Can you work these out from the model? Positions are in its coordinate system, mm. Face numbers are marked on the shaded views. A direction names the side the tool comes from. Coordinates: 2 decimals unless noted, no trailing zeros. Order: outer loops, then holes, each group sorted by start corner. A loop starts at its lowest first (then second) coordinate and runs counter-clockwise, first axis right, second up. Notation, with made-up numbers: (-8.75, -16) -> (-2.75, -16) arc R21 cw to (-2.75, 18) -> close; hole circle Ø1 at (51.5, 2.25). An arc over 180 degrees is marked (long way). Write item = value, one per line.
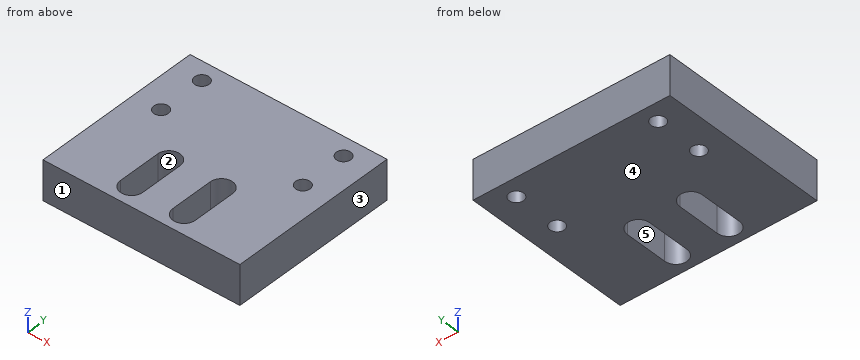
```python
from build123d import *

# Parameters (mm, degrees)
SKETCH1_W           = 75
SKETCH1_H           = 65
SKETCH1_R           = 2.75
BOSS_EXTRUDE1_DEPTH = 15


with BuildPart() as part:
    # Sketch1 → Boss-Extrude1 (new body)
    with BuildSketch(Plane.XY):
        with Locations((0, 1.421243981)):
            Rectangle(SKETCH1_W, SKETCH1_H)
        with Locations((-27, 8.921243981)):
            Circle(SKETCH1_R, mode=Mode.SUBTRACT)
        with Locations((-27, 26.921243981)):
            Circle(SKETCH1_R, mode=Mode.SUBTRACT)
        with Locations((27, 26.921243981)):
            Circle(SKETCH1_R, mode=Mode.SUBTRACT)
        with Locations((27, 8.921243981)):
            Circle(SKETCH1_R, mode=Mode.SUBTRACT)
        with BuildLine():
            Line((-5.75, -7.328756019), (-5.75, -23.828756019))
            ThreePointArc((-5.75, -23.828756019), (-10, -28.078756019), (-14.25, -23.828756019))
            Line((-14.25, -23.828756019), (-14.25, -7.328756019))
            ThreePointArc((-14.25, -7.328756019), (-10, -3.078756019), (-5.75, -7.328756019))
        make_face(mode=Mode.SUBTRACT)
        with BuildLine():
            Line((14.25, -7.328756019), (14.25, -23.828756019))
            ThreePointArc((14.25, -23.828756019), (10, -28.078756019), (5.75, -23.828756019))
            Line((5.75, -23.828756019), (5.75, -7.328756019))
            ThreePointArc((5.75, -7.328756019), (10, -3.078756019), (14.25, -7.328756019))
        make_face(mode=Mode.SUBTRACT)
    extrude(amount=BOSS_EXTRUDE1_DEPTH)


solid = part.part
```
Item 1: I want a section at C-C, the plane x = 27. Please give me the cut outline in (y, z).
A:
outline = (-31.08, 0) -> (6.17, 0) -> (6.17, 15) -> (-31.08, 15) -> close; (11.67, 0) -> (24.17, 0) -> (24.17, 15) -> (11.67, 15) -> close; (29.67, 0) -> (33.92, 0) -> (33.92, 15) -> (29.67, 15) -> close
Item 2: If we mould it in two halves opening along Y, with no side actions, what happens to the marked faces 1, 2 and 3? For each: pulls with the +Y half, pulls with the -Y half, needs draft (parallel to the pull), parting line crosses it, or undercut.
A:
face_1 = pulls with the -Y half
face_2 = undercut
face_3 = needs draft
Item 3: I want a section at D-D, the plane z = 5. Please give me the cut outline in (x, y), plus the area to 3 significant figures.
A:
outline = (-37.5, -31.08) -> (37.5, -31.08) -> (37.5, 33.92) -> (-37.5, 33.92) -> close; hole circle Ø5.5 at (-27, 8.92); hole circle Ø5.5 at (-27, 26.92); hole (-14.25, -23.83) arc R4.25 ccw to (-5.75, -23.83) -> (-5.75, -7.33) arc R4.25 ccw to (-14.25, -7.33) -> close; hole (5.75, -23.83) arc R4.25 ccw to (14.25, -23.83) -> (14.25, -7.33) arc R4.25 ccw to (5.75, -7.33) -> close; hole circle Ø5.5 at (27, 8.92); hole circle Ø5.5 at (27, 26.92)
area = 4,390 mm2
Item 4: I want a section at B-B, the plane y = -23. Please give me the cut outline in (x, z).
A:
outline = (-37.5, 0) -> (-14.25, 0) -> (-14.25, 15) -> (-37.5, 15) -> close; (-5.75, 0) -> (5.75, 0) -> (5.75, 15) -> (-5.75, 15) -> close; (14.25, 0) -> (37.5, 0) -> (37.5, 15) -> (14.25, 15) -> close
Item 5: I want a section at A-A, the plane x = -10. Please give me the cut outline in (y, z), plus the area to 3 significant figures.
A:
outline = (-31.08, 0) -> (-28.08, 0) -> (-28.08, 15) -> (-31.08, 15) -> close; (-3.08, 0) -> (33.92, 0) -> (33.92, 15) -> (-3.08, 15) -> close
area = 600 mm2
Item 6: If I drill on probe 1 along Y at (x, z) = (-27, 5.5); probe 2 along X at (y, z) = (-16, 13.5); probe 3 along X at (y, z) = (-3.5, 5.25), over which ranges is the centre line in solid material (lowest first)?
A:
probe_1 = -31.08 to 6.17, 11.67 to 24.17, 29.67 to 33.92
probe_2 = -37.5 to -14.25, -5.75 to 5.75, 14.25 to 37.5
probe_3 = -37.5 to -11.84, -8.16 to 8.16, 11.84 to 37.5
Item 7: For the marked faces 4 and 5, which set-ups out of +Z, -Z, +X, -X, +Y, -Y let a thin tool reach every point of the face, with its end or its side?
A:
face_4 = -Z, +X, -X, +Y, -Y
face_5 = +Z, -Z
